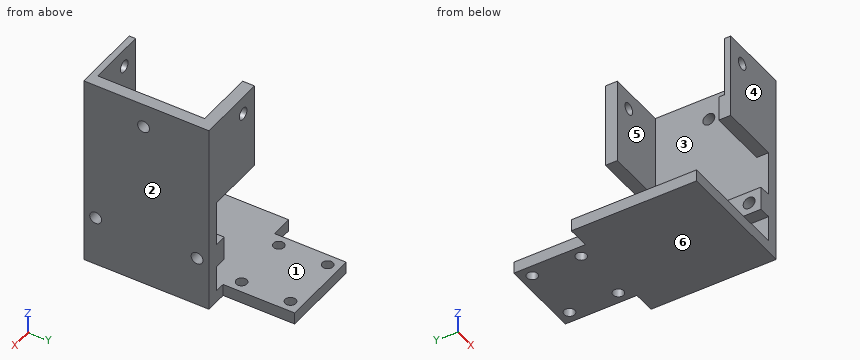
from build123d import *

# Parameters (mm, degrees)
SKETCH1_R               = 2.25
BOSS_EXTRUDE1_DEPTH     = 5
SKETCH2_W               = 52.5
SKETCH2_H               = 52.5
SKETCH2_W_2             = 42.5
SKETCH2_H_2             = 42.5
BOSS_EXTRUDE2_DEPTH     = 40
BOSS_EXTRUDE3_DEPTH     = 36
CUT_EXTRUDE2_DEPTH      = 121.157448791
CUT_EXTRUDE2_DEPTH_BACK = 121.157448791
SKETCH6_R               = 2.5
CUT_EXTRUDE3_DEPTH      = 149.234611343
CUT_EXTRUDE3_DEPTH_BACK = 149.234611343
SKETCH7_R               = 2.5
SKETCH8_W               = 40
SKETCH8_H               = 36.5
CUT_EXTRUDE4_DEPTH      = 24
SKETCH9_W               = 25
SKETCH9_H               = 25.519409936
CUT_EXTRUDE5_DEPTH      = 2.35
SKETCH10_W              = 5
SKETCH10_H              = 30
CUT_EXTRUDE6_DEPTH      = 119
SKETCH11_W              = 40
SKETCH11_H              = 52.5
CUT_EXTRUDE7_DEPTH      = 47.5
SKETCH12_R              = 2.5
CUT_EXTRUDE8_DEPTH      = 119
BOSS_EXTRUDE4_START     = 5
SKETCH13_W              = 10
SKETCH13_H              = 52.5
SKETCH13_R              = 2.5
BOSS_EXTRUDE4_DEPTH     = 5


with BuildPart() as part:
    # Sketch1 → Boss-Extrude1 (new body)
    with BuildSketch(Plane.XY):
        Polygon((0, 30), (-9.25, 30), (-9.25, 82.5), (0, 82.5), (0, 112.5), (34, 112.5), (34, 82.5), (43.25, 82.5), (43.25, 30), (34, 30), (34, 0), (0, 0), align=None)
        with Locations((4.75, 25.25)):
            Circle(SKETCH1_R, mode=Mode.SUBTRACT)
        with Locations((29.25, 25.25)):
            Circle(SKETCH1_R, mode=Mode.SUBTRACT)
        with Locations((29.25, 4.75)):
            Circle(SKETCH1_R, mode=Mode.SUBTRACT)
        with Locations((4.75, 4.75)):
            Circle(SKETCH1_R, mode=Mode.SUBTRACT)
        with Locations((4.75, 107.75)):
            Circle(SKETCH1_R, mode=Mode.SUBTRACT)
        with Locations((29.25, 107.75)):
            Circle(SKETCH1_R, mode=Mode.SUBTRACT)
        with Locations((29.25, 87.25)):
            Circle(SKETCH1_R, mode=Mode.SUBTRACT)
        with Locations((4.75, 87.25)):
            Circle(SKETCH1_R, mode=Mode.SUBTRACT)
    extrude(amount=BOSS_EXTRUDE1_DEPTH)

    # Sketch2 → Boss-Extrude2 (add)
    with BuildSketch(Plane.XY.offset(5)):
        with Locations((17, 56.25)):
            Rectangle(SKETCH2_W, SKETCH2_H)
        with Locations((17, 56.25)):
            Rectangle(SKETCH2_W_2, SKETCH2_H_2, mode=Mode.SUBTRACT)
    extrude(amount=BOSS_EXTRUDE2_DEPTH)

    # Sketch5 → Boss-Extrude3 (add)
    with BuildSketch(Plane.XY.offset(45)):
        Polygon((43.25, 82.5), (43.25, 30), (13.25, 30), (13.25, 35), (38.25, 35), (38.25, 77.5), (13.25, 77.5), (13.25, 82.5), align=None)
    extrude(amount=BOSS_EXTRUDE3_DEPTH)

    # Sketch6 → Cut-Extrude2 (cut, two sides: drawn at the far end of the back side and taken through both)
    with BuildSketch(Plane.XZ.offset(-77.5).offset(-CUT_EXTRUDE2_DEPTH_BACK)):
        with Locations(Location((20.75, 73.5, 0), (0, 0, 270))):
            Circle(SKETCH6_R)
    extrude(amount=CUT_EXTRUDE2_DEPTH + CUT_EXTRUDE2_DEPTH_BACK, mode=Mode.SUBTRACT)

    # Sketch7 → Cut-Extrude3 (cut, two sides: drawn at the far end of the back side and taken through both)
    with BuildSketch(Plane(origin=(43.25, 0, 0), x_dir=(0, 0, -1), z_dir=(1, 0, 0)).offset(-CUT_EXTRUDE3_DEPTH_BACK)):
        with Locations(Location((-71, 55.075, 0), (0, 0, 90))):
            Circle(SKETCH7_R)
    extrude(amount=CUT_EXTRUDE3_DEPTH + CUT_EXTRUDE3_DEPTH_BACK, mode=Mode.SUBTRACT)

    # Sketch8 → Cut-Extrude4 (cut)
    with BuildSketch(Plane.ZY.offset(9.25)):
        with Locations((25, 56.25)):
            Rectangle(SKETCH8_W, SKETCH8_H)
    extrude(amount=-CUT_EXTRUDE4_DEPTH, mode=Mode.SUBTRACT)

    # Sketch9 → Cut-Extrude5 (cut)
    with BuildSketch(Plane(origin=(0, 35, 0), x_dir=(1, 0, 0), z_dir=(0, 1, 0))):
        with Locations((25.75, -68.240295032)):
            Rectangle(SKETCH9_W, SKETCH9_H)
    extrude(amount=-CUT_EXTRUDE5_DEPTH, mode=Mode.SUBTRACT)

    # Sketch10 → Cut-Extrude6 (cut)
    with BuildSketch(Plane.ZY):
        with Locations((2.5, 15)):
            Rectangle(SKETCH10_W, SKETCH10_H)
    extrude(amount=-CUT_EXTRUDE6_DEPTH, mode=Mode.SUBTRACT)

    # Sketch11 → Cut-Extrude7 (cut)
    with BuildSketch(Plane.ZY.offset(9.25)):
        with Locations((25, 56.25)):
            Rectangle(SKETCH11_W, SKETCH11_H)
    extrude(amount=-CUT_EXTRUDE7_DEPTH, mode=Mode.SUBTRACT)

    # Sketch12 → Cut-Extrude8 (cut)
    with BuildSketch(Plane.ZY.offset(-38.25)):
        with Locations(Location((21, 77.5, 0), (0, 0, 270))):
            Circle(SKETCH12_R)
        with Locations(Location((21, 35, 0), (0, 0, 270))):
            Circle(SKETCH12_R)
    extrude(amount=-CUT_EXTRUDE8_DEPTH, mode=Mode.SUBTRACT)

    # Sketch13 → Boss-Extrude4 (add)
    with BuildSketch(Plane.ZY.offset(-38.25).offset(BOSS_EXTRUDE4_START)):
        with Locations((21, 56.25)):
            Rectangle(SKETCH13_W, SKETCH13_H)
        with Locations(Location((21, 77.5, 0), (0, 0, 270))):
            Circle(SKETCH13_R, mode=Mode.SUBTRACT)
        with Locations(Location((21, 35, 0), (0, 0, 270))):
            Circle(SKETCH13_R, mode=Mode.SUBTRACT)
    extrude(amount=-BOSS_EXTRUDE4_DEPTH)


solid = part.part
Here's how the part is built. I have some questions about the finished solid (model axes, mm). Face numbers are marked on the shaded views. A direction names the side the tool comes from. Give positions to 0.01 mm unless a question says otherwise; leave off trailing zeros. Order: outer loops, then holes, each group sorted by start corner. A loop starts at its lowest first (then second) coordinate and runs counter-clockwise, first axis right, second up. Notation, with made-up numbers: (-20.75, 36) -> (-13.75, 36) arc R17 cw to (-13.75, 53) -> close; hole circle Ø7 at (6.25, 38.25). An arc over 180 degrees is marked (long way). Use a Markdown table: item, result. Add a question column.
Item 1: If we mould it in two halves opening along Y, with no side actions, what happens to the marked faces 3, 4, 5 and 6? For each: pulls with the +Y half, pulls with the -Y half, needs draft (parallel to the pull), parting line crosses it, or undercut.
Item 2: Imagine slicing it at A-A on x = 36. Please give me the cut outline in (y, z), plus the area to 3 significant figures.
Item 3: Imagine slicing it at D-D on x = 20.75. Please give me the cut outline in (y, z).
Item 4: I need wall thicknesses on line 1 (X direction, y = 79.6, z = 73.5); line 2 (Y direction, x = 30.5, z = 50.5); line 3 (Z direction, x = 27.5, y = 82). Which ranges of each line are inside material? Lowest first, please.
Item 5: Will these pins go through, and if not, where does the flat tip stop? pin 1 (1.5 mm diameter, centred on x = 27, y = 100, fed in from +Z); pin 2 (5.5 mm diameter, centred on y = 93, z = 3, fed in from -X); pin 3 (8 mm diameter, centred on y = 61, z = 23.5, fed in from -X).
Item 6: Imagine slicing it at C-C on z = 65. Please give me the cut outline in (x, y), plus the area to 3 significant figures.
Item 7: Imagine slicing it at B-B on y = 87.25. Please give me the cut outline in (x, z), plus the area to 3 significant figures.
Item 8: For the marked faces 1 and 2, which set-ups out of +Z, -Z, +X, -X, +Y, -Y let a thin tool reach every point of the face, with its end or its side?
Data:
| question | item | result |
|---|---|---|
| 1 | face 3 | undercut |
| 1 | face 4 | pulls with the -Y half |
| 1 | face 5 | undercut |
| 1 | face 6 | needs draft |
| 2 | outline | (30, 0) -> (82.5, 0) -> (82.5, 5) -> (30, 5) -> close; (30, 16) -> (82.5, 16) -> (82.5, 26) -> (30, 26) -> close; (30, 45) -> (35, 45) -> (35, 55.48) -> (32.65, 55.48) -> (32.65, 81) -> (30, 81) -> close; (77.5, 45) -> (82.5, 45) -> (82.5, 81) -> (77.5, 81) -> close; hole circle Ø5 at (35, 21); hole circle Ø5 at (77.5, 21) |
| 2 | area | 1,050 mm² |
| 3 | outline | (30, 0) -> (112.5, 0) -> (112.5, 5) -> (30, 5) -> close; (30, 45) -> (35, 45) -> (35, 55.48) -> (32.65, 55.48) -> (32.65, 71) -> (30, 71) -> close; (30, 76) -> (32.65, 76) -> (32.65, 81) -> (30, 81) -> close; (77.5, 45) -> (82.5, 45) -> (82.5, 71) -> (77.5, 71) -> close; (77.5, 76) -> (82.5, 76) -> (82.5, 81) -> (77.5, 81) -> close |
| 4 | line 1 | x = 13.25 to 18.25, 23.25 to 43.25 |
| 4 | line 2 | y = 30 to 35, 77.5 to 82.5 |
| 4 | line 3 | z = 0 to 5, 45 to 81 |
| 5 | pin 1 | stops at z = 5 |
| 5 | pin 2 | stops at x = 0 |
| 5 | pin 3 | stops at x = 33.25 |
| 6 | outline | (13.25, 30) -> (43.25, 30) -> (43.25, 82.5) -> (13.25, 82.5) -> (13.25, 77.5) -> (38.25, 77.5) -> (38.25, 32.65) -> (13.25, 32.65) -> close |
| 6 | area | 454 mm² |
| 7 | outline | (0, 0) -> (2.5, 0) -> (2.5, 5) -> (0, 5) -> close; (7, 0) -> (27, 0) -> (27, 5) -> (7, 5) -> close; (31.5, 0) -> (34, 0) -> (34, 5) -> (31.5, 5) -> close |
| 7 | area | 125 mm² |
| 8 | face 1 | -X, +Y, -Y |
| 8 | face 2 | +Z, -Z, +X, +Y, -Y |
